Design review of the part built by this model. Coordinates are the model's own, in mm. A direction names the side the tool comes from. Round coordinates to 2 decimals unless told otherwise and drop trailing zeros. Order: outer loops, then holes, each group sorted by start corner. A loop starts at its lowest first (then second) coordinate and runs counter-clockwise, first axis right, second up. Notation, with made-up numbers: M 37.25,39.5 L 79.25,39.5 A19 ccw 79.25,56.5 Z; hole C 29.5,68 d7. An arc over 180 degrees is marked long. Use a Markdown table: item, result. Add a question column.
(1) To check wall thickness, follow probe 1 along Y at (x, z) = (-12.5, 1); probe 2 along X at (y, z) = (15, 1.75); probe 3 along X at (y, z) = (27.5, 5.75). State the ranges of each line that lie inside material, in increasing order. Write a range as from..to.
(2) Take a section at C-C (y = 2.5). Write out the cut boundary in (x, z).
(3) Take a section at B-B (x = -11.5). Write out the cut boundary in (y, z), then the cut area to 3 significant figures.
(4) The part is to be moulded in two halves that separate along X. For faces 5 (the face through (36.5, -27, 9.1)), 6 (the face through (-41.188, 31.785, 11.066)), 7 (the face through (44, -3.5, 1)), say which applies: released by +X, released by -X, zero draft, split by the parting line, or undercut.
(5) Machinability: for faces 1 (the face through (-1, 33, 5)), 2 (the face through (11, 34, 4.12)), 3 (the face through (-37, -26, 0)), 4 (the face through (32.564, -25.691, 10.57)), which of the approach directions +Z, -Z, +X, -X, +Y, -Y give a long, thin tool a straight path to every point of the face, cutting with its end or side? Answer none if there is none.
(6) Take a section at A-A (z = 6.25). Count the separate pieces of the cut face and the enclosed holes in it, then the cut area to 3 significant figures.
(7) For pin 1 (1.6 mm diameter, centred on x = -44, y = 1, fed in from -Z); pin 2 (2 mm diameter, centred on x = 43.5, y = -12, fed in from -Z); pin 3 (1 mm diameter, centred on y = 34.5, z = 2.5, fed in from +X), all flat-tipped, find the tip position at first contact; note any pin that passes through.
```python
from build123d import *

# Parameters (mm, degrees)
SKETCH_1_W                     = 89
SKETCH_1_H                     = 70
EXTRUDE_1_DEPTH                = 12
FILLET_1_R                     = 7.7
CHAMFER_1_SIZE                 = 2.36
SHELL_1_T                      = -2
CUT_EXTRUDE_1_REACH            = 72
SKETCH_2_W                     = 9.92
SKETCH_2_H                     = 4.12
SKETCH_2_W_2                   = 9.17
SKETCH_2_H_2                   = 2.37
SKETCH_2_W_3                   = 12.93
SKETCH_2_H_3                   = 2.54
CUT_EXTRUDE_2_REACH            = 91
SKETCH_3_W                     = 2.54
SKETCH_3_H                     = 12.93
SKETCH_3_W_2                   = 4
SKETCH_3_H_2                   = 17
CUT_EXTRUDE_3_REACH            = 91
SKETCH_4_W                     = 2.54
SKETCH_4_H                     = 12.93
SKETCH_5_R                     = 4.5
EXTRUDE_2_DEPTH                = 10
HOLE_WIZARD_M2_5_1_D           = 2.9
HOLE_WIZARD_M2_5_1_CBORE_D     = 5.5
HOLE_WIZARD_M2_5_1_CBORE_DEPTH = 2.9


with BuildPart() as part:
    # 草圖1 → 填料-伸長1 (new body)
    with BuildSketch(Plane.XY):
        Rectangle(SKETCH_1_W, SKETCH_1_H)
    extrude(amount=EXTRUDE_1_DEPTH)

    # 圓角1
    fillet_1_edges = [part.edges().sort_by_distance(p)[0] for p in [
        (44.5, -35, 6),
        (-44.5, -35, 6),
        (-44.5, 35, 6),
        (44.5, 35, 6),
    ]]
    fillet(fillet_1_edges, radius=FILLET_1_R)

    # 導角1
    chamfer_1_edges = [part.edges().sort_by_distance(p)[0] for p in [
        (0, -35, 12),
        (-44.5, 0, 12),
        (44.5, 0, 12),
        (0, 35, 12),
        (-42.244722215, 32.744722215, 12),
        (42.244722215, 32.744722215, 12),
        (42.244722215, -32.744722215, 12),
        (-42.244722215, -32.744722215, 12),
    ]]
    chamfer(chamfer_1_edges, length=CHAMFER_1_SIZE)

    # 薄殼1
    shell_1_openings = [part.faces().sort_by_distance(p)[0] for p in [
        (0, 0, 0),
    ]]
    offset(amount=SHELL_1_T, openings=shell_1_openings, kind=Kind.INTERSECTION)

    # 草圖2 → 除料-伸長1 (cut, up to next)
    with BuildSketch(Plane(origin=(0, 35, 0), x_dir=(1, 0, 0), z_dir=(0, 1, 0)), mode=Mode.PRIVATE) as cut_extrude_1_sk1:
        with Locations((11.53, -2.06)):
            Rectangle(SKETCH_2_W, SKETCH_2_H)
    cut_extrude_1_tool1 = extrude(cut_extrude_1_sk1.sketch, amount=-CUT_EXTRUDE_1_REACH, mode=Mode.PRIVATE) & part.part
    add(cut_extrude_1_tool1.solids().sort_by_distance((11.53, 35, 2.06))[0], mode=Mode.SUBTRACT)
    # 草圖2 → 除料-伸長1 (cut, up to next)
    with BuildSketch(Plane(origin=(0, 35, 0), x_dir=(1, 0, 0), z_dir=(0, 1, 0)), mode=Mode.PRIVATE) as cut_extrude_1_sk2:
        with Locations((-3.085, -1.185)):
            Rectangle(SKETCH_2_W_2, SKETCH_2_H_2)
    cut_extrude_1_tool2 = extrude(cut_extrude_1_sk2.sketch, amount=-CUT_EXTRUDE_1_REACH, mode=Mode.PRIVATE) & part.part
    add(cut_extrude_1_tool2.solids().sort_by_distance((-3.085, 35, 1.185))[0], mode=Mode.SUBTRACT)
    # 草圖2 → 除料-伸長1 (cut, up to next)
    with BuildSketch(Plane(origin=(0, 35, 0), x_dir=(1, 0, 0), z_dir=(0, 1, 0)), mode=Mode.PRIVATE) as cut_extrude_1_sk3:
        with Locations((-19.895, -1.27)):
            Rectangle(SKETCH_2_W_3, SKETCH_2_H_3)
    cut_extrude_1_tool3 = extrude(cut_extrude_1_sk3.sketch, amount=-CUT_EXTRUDE_1_REACH, mode=Mode.PRIVATE) & part.part
    add(cut_extrude_1_tool3.solids().sort_by_distance((-19.895, 35, 1.27))[0], mode=Mode.SUBTRACT)

    # 草圖3 → 除料-伸長2 (cut, up to next)
    with BuildSketch(Plane(origin=(44.5, 0, 0), x_dir=(0, 0, -1), z_dir=(1, 0, 0)), mode=Mode.PRIVATE) as cut_extrude_2_sk1:
        with Locations((-1.27, 2.965)):
            Rectangle(SKETCH_3_W, SKETCH_3_H)
    cut_extrude_2_tool1 = extrude(cut_extrude_2_sk1.sketch, amount=-CUT_EXTRUDE_2_REACH, mode=Mode.PRIVATE) & part.part
    add(cut_extrude_2_tool1.solids().sort_by_distance((44.5, 2.965, 1.27))[0], mode=Mode.SUBTRACT)
    # 草圖3 → 除料-伸長2 (cut, up to next)
    with BuildSketch(Plane(origin=(44.5, 0, 0), x_dir=(0, 0, -1), z_dir=(1, 0, 0)), mode=Mode.PRIVATE) as cut_extrude_2_sk2:
        with Locations((-2, -15)):
            Rectangle(SKETCH_3_W_2, SKETCH_3_H_2)
    cut_extrude_2_tool2 = extrude(cut_extrude_2_sk2.sketch, amount=-CUT_EXTRUDE_2_REACH, mode=Mode.PRIVATE) & part.part
    add(cut_extrude_2_tool2.solids().sort_by_distance((44.5, -15, 2))[0], mode=Mode.SUBTRACT)

    # 草圖4 → 除料-伸長3 (cut, up to next)
    with BuildSketch(Plane.ZY.offset(44.5), mode=Mode.PRIVATE) as cut_extrude_3_sk1:
        with Locations((1.27, 1.535)):
            Rectangle(SKETCH_4_W, SKETCH_4_H)
    cut_extrude_3_tool1 = extrude(cut_extrude_3_sk1.sketch, amount=-CUT_EXTRUDE_3_REACH, mode=Mode.PRIVATE) & part.part
    add(cut_extrude_3_tool1.solids().sort_by_distance((-44.5, 1.535, 1.27))[0], mode=Mode.SUBTRACT)

    # 草圖5 → 填料-伸長2 (add)
    with BuildSketch(Plane(origin=(0, 0, 10), x_dir=(-1, 0, 0), z_dir=(0, 0, -1))):
        with Locations((-35.311572875, 25.811572875)):
            Circle(SKETCH_5_R)
        with Locations((35.311572875, 25.811572875)):
            Circle(SKETCH_5_R)
        with Locations((35.311572875, -25.811572875)):
            Circle(SKETCH_5_R)
        with Locations((-35.311572875, -25.811572875)):
            Circle(SKETCH_5_R)
    extrude(amount=EXTRUDE_2_DEPTH)

    # M2.5 六角承窩頭蓋螺釘的柱孔1 (through all)
    with Locations(Plane(origin=(35.311572875, -25.811572875, 12), x_dir=(1, 0, 0), z_dir=(0, 0, 1))):
        with Locations((0, 0), (-70.62314575, 0), (-70.62314575, 51.62314575), (0, 51.62314575)):
            CounterBoreHole(HOLE_WIZARD_M2_5_1_D / 2, HOLE_WIZARD_M2_5_1_CBORE_D / 2, HOLE_WIZARD_M2_5_1_CBORE_DEPTH)


solid = part.part
```
Verdict:
| question | item | result |
|---|---|---|
| 1 | probe 1 | y = -35..-33, 33..35 |
| 1 | probe 2 | x = -44.5..-42.5, 42.5..44.5 |
| 1 | probe 3 | x = -44.5..-42.5, -39.48..-31.14, 31.14..39.48, 42.5..44.5 |
| 2 | outline | M -44.5,2.54 L -42.5,2.54 L -42.5,8.81 L -41.31,10 L 41.31,10 L 42.5,8.81 L 42.5,2.54 L 44.5,2.54 L 44.5,9.64 L 42.14,12 L -42.14,12 L -44.5,9.64 Z |
| 3 | outline | M -35,0 L -33,0 L -33,8.81 L -31.81,10 L 31.81,10 L 33,8.81 L 33,0 L 35,0 L 35,9.64 L 32.64,12 L -32.64,12 L -35,9.64 Z |
| 3 | area | 176 mm^2 |
| 4 | face 5 | undercut |
| 4 | face 6 | released by -X |
| 4 | face 7 | zero draft |
| 5 | face 1 | -Z |
| 5 | face 2 | -Z, +Y |
| 5 | face 3 | -Z, +X, -X, +Y, -Y |
| 5 | face 4 | +Z |
| 6 | separate pieces | 5 |
| 6 | enclosed holes | 5 |
| 6 | area | 825 mm^2 |
| 7 | pin 1 | stops at z = 2.54 |
| 7 | pin 2 | stops at z = 4 |
| 7 | pin 3 | stops at x = 40.59 |
